```python
from build123d import *

# Parameters (mm, degrees)
CYLINDER032_R             = 12.5
CYLINDER032_DEPTH         = 35
CYLINDER030_R             = 16
CYLINDER030_DEPTH         = 10
CYLINDER033_R             = 7
CYLINDER033_DEPTH         = 2
CYLINDER034_R             = 14
CYLINDER034_DEPTH         = 2
CYLINDER031_R             = 2
CYLINDER031_DEPTH         = 10
CYLINDER031_ROLL_ANGLE    = 90
ARRAY004_X_COUNT          = 2
ARRAY004_X_PITCH          = 36
BOX014_W                  = 44
BOX014_H                  = 5
BOX014_DEPTH              = 10
POCKET_DEPTH              = 8
FUSION026_PLACEMENT_ANGLE = 180


with BuildPart() as cylinder032:
    # Cylinder032 → Cylinder032 (new body)
    with BuildSketch(Plane.XY):
        Circle(CYLINDER032_R)
    extrude(amount=CYLINDER032_DEPTH)


with BuildPart() as cuerpo_arandela001:
    # Cylinder030 → Cylinder030 (new body)
    with BuildSketch(Plane.XY):
        Circle(CYLINDER030_R)
    extrude(amount=CYLINDER030_DEPTH)

    # Cut004024: cut Cylinder032
    add(cylinder032.part, mode=Mode.SUBTRACT)


with BuildPart() as cylinder033:
    # Cylinder033 → Cylinder033 (new body)
    with BuildSketch(Plane.XY):
        Circle(CYLINDER033_R)
    extrude(amount=CYLINDER033_DEPTH)


with BuildPart() as tapa_arandela001:
    # Cylinder034 → Cylinder034 (new body)
    with BuildSketch(Plane.XY):
        Circle(CYLINDER034_R)
    extrude(amount=CYLINDER034_DEPTH)

    # Cut004025: cut Cylinder033
    add(cylinder033.part, mode=Mode.SUBTRACT)


with BuildPart() as array004:
    # Cylinder031 → Cylinder031 (new body)
    with BuildSketch(Plane.XY):
        Circle(CYLINDER031_R)
    extrude(amount=CYLINDER031_DEPTH)


with BuildPart() as array004_1:
    # Cylinder031 roll: moved
    add(array004.part.rotate(Axis((0, 0, 0), (1, 0, 0)), CYLINDER031_ROLL_ANGLE))


with BuildPart() as array004_2:
    # Cylinder031 placement: moved
    add(array004_1.part.moved(Location((18, 8, 5))))

    # Array004 X: Array004 ×2


with BuildPart() as array004_3:
    add(array004_2.part)
    with Locations(*[(-i * ARRAY004_X_PITCH, 0, 0) for i in range(1, ARRAY004_X_COUNT)]):
        add(array004_2.part)


with BuildPart() as porta_rodamiento_grande:
    # Box014 → Box014 (new body)
    with BuildSketch(Plane(origin=(-22, 0, 0), x_dir=(1, 0, 0), z_dir=(0, 0, 1))):
        with Locations((22, 2.5)):
            Rectangle(BOX014_W, BOX014_H)
    extrude(amount=BOX014_DEPTH)

    # Cut004026: cut Array004
    add(array004_3.part, mode=Mode.SUBTRACT)


with BuildPart() as porta_rodamiento_grande_1:
    # Cut004026 placement: moved
    add(porta_rodamiento_grande.part.moved(Location((0, 11, 0))))

    # Sketch001 → Pocket (cut)
    with BuildSketch(Plane(origin=(0, 11, 10), x_dir=(1, 0, 0), z_dir=(0, 0, 1))):
        with BuildLine():
            ThreePointArc((5.937171, 0), (0, 1.5), (-5.937171, 0))
            Line((-5.937171, 0), (5.937171, 0))
        make_face()
    extrude(amount=-POCKET_DEPTH, mode=Mode.SUBTRACT)

    # Fusion026: union cuerpo-arandela001, tapa-arandela001
    add(cuerpo_arandela001.part)
    add(tapa_arandela001.part)


with BuildPart() as porta_rodamiento_grande_2:
    # Fusion026 placement: moved
    add(porta_rodamiento_grande_1.part.moved(Location((-30, 51, 47))).rotate(Axis((-30, 51, 47), (1, 0, 0)), FUSION026_PLACEMENT_ANGLE))


solid = porta_rodamiento_grande_2.part
```
Design review of the part built by this model. Coordinates are the model's own, in mm. A direction names the side the tool comes from. Give positions to 0.01 mm unless a question says otherwise; leave off trailing zeros. Order: outer loops, then holes, each group sorted by start corner. A loop starts at its lowest first (then second) coordinate and runs counter-clockwise, first axis right, second up. Notation, with made-up numbers: (48, 54.5) - (56, 54.5) arc R22 cw to (56, 68.5) - close; hole circle Ø2 at (13.5, 47). An arc over 180 degrees is marked (long way). Use a Markdown table: item, result. Add a question column.
(1) Wall thickness on probe 1 along Y at (x, z) = (-30, 45.7); probe 2 along X at (y, z) = (51, 45.9); probe 3 along X at (y, z) = (51, 40.5): over which ranges is each line inside the solid? List them lowest first. Write a range as [from, to].
(2) Add section D-D on z = 44.5. Give the boundary of the cut face in (x, y).
(3) Mouldability with a two-part tool opening along X and no side actions: class faces 1 (the face through (-48, 37, 44)), 2 (the face through (-8, 38, 42)), 3 (the face through (-45.7, 40, 42.1)), 4 (the face through (-52, 38, 42)) as +X half, -X half, draft (parallel to the pull), parting line (faces both ways), or undercut.
(4) Add section B-B on y = 51. Give the boundary of the cut face in (x, z).
(5) Machinability: for faces 5 (the face through (-24.6, 56.4, 45)), 6 (the face through (-12, 37, 44)), 7 (the face through (-14.4, 40, 42.1)), which of the approach directions +Z, -Z, +X, -X, +Y, -Y give a long, thin tool a straight path to every point of the face, cutting with its end or side? Answer none if there is none.
(6) Add section A-A on z = 42. Give the boundary of the cut face in (x, y), then the cut area to 3 significant figures.
(7) Add section C-C on x = -12. Give the boundary of the cut face in (y, z).
(8) Clearance check with flat-ended pins moving along their axes: P1, Ø5, axis at x = -48, z = 42, coming from the -Y side; P2, Ø2, axis at x = -42.5, z = 38.5, coming from the +Y side; P3, Ø2, axis at y = 48, z = 38, coming from the +X side; P4, Ø2, axis at y = 60, z = 39, coming from the +X side. State where each tip first meets the part, or that it passes through.
Report:
| question | item | result |
|---|---|---|
| 1 | probe 1 | y = [35, 44], [58, 67] |
| 1 | probe 2 | x = [-46, -37], [-23, -14] |
| 1 | probe 3 | x = [-46, -42.5], [-17.5, -14] |
| 2 | outline | (-52, 35) - (-8, 35) - (-8, 40) - (-18.38, 40) arc R16 ccw (long way) to (-41.62, 40) - (-52, 40) - close; hole circle Ø25 at (-30, 51) |
| 3 | face 1 | undercut |
| 3 | face 2 | +X half |
| 3 | face 3 | draft |
| 3 | face 4 | -X half |
| 4 | outline | (-46, 37) - (-42.5, 37) - (-42.5, 45) - (-37, 45) - (-37, 47) - (-46, 47) - close; (-23, 45) - (-17.5, 45) - (-17.5, 37) - (-14, 37) - (-14, 47) - (-23, 47) - close |
| 5 | face 5 | -Z |
| 5 | face 6 | +Y, -Y |
| 5 | face 7 | +Z, -Z, +X |
| 6 | outline | (-52, 35) - (-50, 35) - (-50, 40) - (-52, 40) - close; (-46, 35) - (-14, 35) - (-14, 40) - (-18.38, 40) arc R16 ccw (long way) to (-41.62, 40) - (-46, 40) - close; (-10, 35) - (-8, 35) - (-8, 40) - (-10, 40) - close; hole circle Ø25 at (-30, 51) |
| 6 | area | 413 mm² |
| 7 | outline | (35, 37) - (40, 37) - (40, 40) - (35, 40) - close; (35, 44) - (40, 44) - (40, 47) - (35, 47) - close |
| 8 | P1 | stops at y = 35 |
| 8 | P2 | stops at y = 62.12 |
| 8 | P3 | stops at x = -14.13 |
| 8 | P4 | stops at x = -16.14 |
